Build history of the part. All positions in model axes, mm. Round coordinates to 2 decimals unless told otherwise and drop trailing zeros. Order: outer loops, then holes, each group sorted by start corner. A loop starts at its lowest first (then second) coordinate and runs counter-clockwise, first axis right, second up. Notation, with made-up numbers: M 38,-27 L 47,-27 A23 ccw 47,-3 Z; hole C -37.5,-23 d8. An arc over 180 degrees is marked long. One line per question, with ' | ' between items. Start each with the question number.
from build123d import *

# Parameters (mm, degrees)
F0_W     = 82.2
F0_H     = 62.4
F0_R     = 1.5
F0_R_2   = 9.4
F0_R_3   = 2
F0_R_4   = 3
F1_DEPTH = 4
F2_R     = 3


with BuildPart() as f1:
    # F0 (on Front) → F1 (new body)
    with BuildSketch(Plane.XZ):
        with Locations((29.7, 19.8)):
            Rectangle(F0_W, F0_H)
        with Locations((-8.630646, -8.630646)):
            Circle(F0_R, mode=Mode.SUBTRACT)
        Circle(F0_R_2, mode=Mode.SUBTRACT)
        with Locations((9.9, -8.425556)):
            Circle(F0_R_3, mode=Mode.SUBTRACT)
        with Locations((19.8, 0)):
            Circle(F0_R_2, mode=Mode.SUBTRACT)
        with Locations((-8.630646, 9.9)):
            Circle(F0_R, mode=Mode.SUBTRACT)
        with Locations((9.9, 9.9)):
            Circle(F0_R_4, mode=Mode.SUBTRACT)
        with Locations((29.7, -8.425556)):
            Circle(F0_R_3, mode=Mode.SUBTRACT)
        with Locations((49.5, -8.425556)):
            Circle(F0_R_3, mode=Mode.SUBTRACT)
        with Locations((39.6, 0)):
            Circle(F0_R_2, mode=Mode.SUBTRACT)
        with Locations((68.030646, -8.630646)):
            Circle(F0_R, mode=Mode.SUBTRACT)
        with Locations((59.4, 0)):
            Circle(F0_R_2, mode=Mode.SUBTRACT)
        with Locations((29.7, 9.9)):
            Circle(F0_R_4, mode=Mode.SUBTRACT)
        with Locations((49.5, 9.9)):
            Circle(F0_R_4, mode=Mode.SUBTRACT)
        with Locations((68.030646, 9.9)):
            Circle(F0_R, mode=Mode.SUBTRACT)
        with Locations((0, 19.8)):
            Circle(F0_R_2, mode=Mode.SUBTRACT)
        with Locations((-8.630646, 29.7)):
            Circle(F0_R, mode=Mode.SUBTRACT)
        with Locations((19.8, 19.8)):
            Circle(F0_R_2, mode=Mode.SUBTRACT)
        with Locations((9.9, 29.7)):
            Circle(F0_R_4, mode=Mode.SUBTRACT)
        with Locations((0, 39.6)):
            Circle(F0_R_2, mode=Mode.SUBTRACT)
        with Locations((-8.630646, 48.230646)):
            Circle(F0_R, mode=Mode.SUBTRACT)
        with Locations((19.8, 39.6)):
            Circle(F0_R_2, mode=Mode.SUBTRACT)
        with Locations((9.9, 48.025556)):
            Circle(F0_R_3, mode=Mode.SUBTRACT)
        with Locations((39.6, 19.8)):
            Circle(F0_R_2, mode=Mode.SUBTRACT)
        with Locations((29.7, 29.7)):
            Circle(F0_R_4, mode=Mode.SUBTRACT)
        with Locations((49.5, 29.7)):
            Circle(F0_R_4, mode=Mode.SUBTRACT)
        with Locations((59.4, 19.8)):
            Circle(F0_R_2, mode=Mode.SUBTRACT)
        with Locations((68.030646, 29.7)):
            Circle(F0_R, mode=Mode.SUBTRACT)
        with Locations((39.6, 39.6)):
            Circle(F0_R_2, mode=Mode.SUBTRACT)
        with Locations((29.7, 48.025556)):
            Circle(F0_R_3, mode=Mode.SUBTRACT)
        with Locations((49.5, 48.025556)):
            Circle(F0_R_3, mode=Mode.SUBTRACT)
        with Locations((59.4, 39.6)):
            Circle(F0_R_2, mode=Mode.SUBTRACT)
        with Locations((68.030646, 48.230646)):
            Circle(F0_R, mode=Mode.SUBTRACT)
    extrude(amount=F1_DEPTH)

    # F2
    f2_edges = [f1.edges().sort_by_distance(p)[0] for p in [
        (70.8, -2, 51),
        (-11.4, -2, 51),
        (-11.4, -2, -11.4),
        (70.8, -2, -11.4),
    ]]
    fillet(f2_edges, radius=F2_R)


solid = f1.part
Item 1: Cut at B-B on z = 39.6. Write the cut outline in (x, y), then the cut area to 3 significant figures.
Item 2: Cut at A-A on x = 19.8. Write the cut outline in (y, z).
Item 3: Wall check: line 1 along Z through (x, y) = (49.5, -1.25); line 2 along X through (y, z) = (-1.8, 0.5); line 3 along Z through (x, y) = (19.8, -3). Give the ranges that are in metal, low to high. Write a range as [from, to].
Item 4: Two-plate mould, pull along X, no slides. Class faces 1 (the face through (70.8, -2, 19)), 2 (the face through (-10.54, -2.03, 50.1)), 3 (the face through (29, -2, -11.4)), 4 (the face through (47.29, -1.97, 31.73)): +X half, -X half, draft (parallel to the pull), parting line (faces both ways), or undercut.
Item 5: Cut at C-C on y = -2.3. Count the separate pieces of the cut face and the enclosed holes in it, then the cut area to 3 significant figures.
Item 6: Flat gauge pins, fed straight in: pin 1 (1.8 mm diameter, centred on x = 68.03, z = -8.63, fed in from -Y); pin 2 (24.5 mm diameter, centred on x = 59.4, z = 39.6, fed in from -Y). Where does each tip first touch, or does it go through?
Item 7: Cut at D-D on x = -0.5. Write the cut outline in (y, z), then the cut area to 3 significant figures.
Results found:
1) outline: M -11.4,-4 L -9.4,-4 L -9.4,0 L -11.4,0 Z; M 9.4,-4 L 10.4,-4 L 10.4,0 L 9.4,0 Z; M 29.2,-4 L 30.2,-4 L 30.2,0 L 29.2,0 Z; M 49,-4 L 50,-4 L 50,0 L 49,0 Z; M 68.8,-4 L 70.8,-4 L 70.8,0 L 68.8,0 Z | area: 28.0 mm^2
2) outline: M -4,-11.4 L 0,-11.4 L 0,-9.4 L -4,-9.4 Z; M -4,9.4 L 0,9.4 L 0,10.4 L -4,10.4 Z; M -4,29.2 L 0,29.2 L 0,30.2 L -4,30.2 Z; M -4,49 L 0,49 L 0,51 L -4,51 Z
3) line 1: z = [-11.4, -10.43], [-6.43, 6.9], [12.9, 26.7], [32.7, 46.03], [50.03, 51] | line 2: x = [-11.4, -9.39], [9.39, 10.41], [29.19, 30.21], [48.99, 50.01], [68.79, 70.8] | line 3: z = [-11.4, -9.4], [9.4, 10.4], [29.2, 30.2], [49, 51]
4) face 1: +X half | face 2: -X half | face 3: draft | face 4: undercut
5) separate pieces: 1 | enclosed holes: 32 | area: 1,490 mm^2
6) pin 1: passes through | pin 2: stops at y = -4
7) outline: M -4,-11.4 L 0,-11.4 L 0,-9.39 L -4,-9.39 Z; M -4,9.39 L 0,9.39 L 0,10.41 L -4,10.41 Z; M -4,29.19 L 0,29.19 L 0,30.21 L -4,30.21 Z; M -4,48.99 L 0,48.99 L 0,51 L -4,51 Z | area: 24.3 mm^2
